Model file for the job. Use its own axes, mm. Round coordinates to 2 decimals unless told otherwise and drop trailing zeros. Order: outer loops, then holes, each group sorted by start corner. A loop starts at its lowest first (then second) coordinate and runs counter-clockwise, first axis right, second up. Notation, with made-up numbers: (30.5, 48) - (39.5, 48) arc R17 ccw to (39.5, 76) - close; hole circle Ø1 at (7.25, 87). An arc over 180 degrees is marked (long way). Use one line per item in the form item = value.
from build123d import *

# Parameters (mm, degrees)
SKETCH1_W            = 25.4
SKETCH1_H            = 50.8
BOSS_EXTRUDE1_DEPTH  = 9.398
LPATTERN1_COUNT      = 2
LPATTERN1_PITCH      = 44.45
LPATTERN1_COUNT_DIR2 = 2
LPATTERN1_PITCH_DIR2 = 19.05


with BuildPart() as part:
    # Sketch1 → Boss-Extrude1 (new body)
    with BuildSketch(Plane.XY):
        Rectangle(SKETCH1_W, SKETCH1_H)
    extrude(amount=BOSS_EXTRUDE1_DEPTH)

    # Sketch3 → #8 Clearance Hole1 (revolve, cut)
    with BuildSketch(Plane(origin=(-9.525, -22.225, 9.398), x_dir=(0, -1, 0), z_dir=(1, 0, 0))):
        Polygon((0, 0), (0, 9.398), (2.54, 9.398), (2.2479, 9.222488613), (2.2479, 0.175511387), (2.54, 0), align=None)
    f_8_clearance_hole1 = revolve(axis=Axis((-9.525, -22.225, 15.748), (0, 0, -1)), mode=Mode.SUBTRACT)

    # LPattern1: 8 Clearance Hole1 2 × 2
    with Locations(*[(j * LPATTERN1_PITCH_DIR2, i * LPATTERN1_PITCH, 0) for i in range(LPATTERN1_COUNT) for j in range(LPATTERN1_COUNT_DIR2) if (i, j) != (0, 0)]):
        add(f_8_clearance_hole1, mode=Mode.SUBTRACT)


solid = part.part
(1) Probe probe 1 along X at (y, z) = (-20.5, 1.5); probe 2 along Y at (x, z) = (-10.5, 7); probe 3 along X at (y, z) = (-23, 6.25). List the from-to ranges inside material, lowest first. Write a range as [from, to].
Report:
probe_1 = [-12.7, -10.97], [-8.08, 8.08], [10.97, 12.7]
probe_2 = [-25.4, -24.25], [-20.2, 20.2], [24.25, 25.4]
probe_3 = [-12.7, -11.64], [-7.41, 7.41], [11.64, 12.7]
(2) Pull direction X, two halves, no side cores. Call faces 1 (the face through (12.7, 0, 5)), 2 (the face through (-11.044, -20.568, 4.762)), 3 (the face through (0, 0, 9.398)): released by +X, released by -X, zero draft, split by the parting line, or undercut.
Report:
face_1 = released by +X
face_2 = undercut
face_3 = zero draft
(3) Pin check, flat tips, straight feed: pin 1 (3.5 mm diameter, centred on x = 9.525, y = 22.225, fed in from -Z); pin 2 (6 mm diameter, centred on x = -9.525, y = 22.225, fed in from +Z). Stop position of each tip, or through.
Report:
pin_1 = through
pin_2 = 9.4
(4) Slice it at A-A on z = 6.5. Give the cut face in (x, y) (3 decimals).
Report:
outline = (-12.7, -25.4) - (12.7, -25.4) - (12.7, 25.4) - (-12.7, 25.4) - close; hole circle Ø4.496 at (-9.525, -22.225); hole circle Ø4.496 at (-9.525, 22.225); hole circle Ø4.496 at (9.525, -22.225); hole circle Ø4.496 at (9.525, 22.225)
(5) Slice it at B-B on y = -20.5. Count the separate pieces of the cut face and the enclosed holes in it, then the cut area to 3 significant figures.
Report:
separate_pieces = 3
enclosed_holes = 0
area = 184 mm2
